The model under review builds one solid part; all positions refer to its coordinate system, in mm. A direction names the side the tool comes from. Give positions to 0.01 mm unless a question says otherwise; leave off trailing zeros. Loops run counter-clockwise (first coordinate to the right, second up) from the corner with the lowest first, then second, coordinate; pieces in that order, holes last. Notation, with made-up numbers: M 69.5,-2 L 123.5,-2 A36 ccw 123.5,35 Z; hole C 74,18 d5. An arc over 180 degrees is marked long. One line per item, written item: value. Start each with the question number.
Q1. For pin 1 (2 mm diameter, centred on x = 67.5, y = 268.5, fed in from +Z); pin 2 (8 mm diameter, centred on x = -8, y = 122.5, fed in from -Z), all flat-tipped, find the tip position at first contact; note any pin that passes through.
Q2. Mouldability with a two-part tool opening along X and no side actions: class faces 3 (the face through (-289, -6, 10)), 4 (the face through (288, -6, 10)), 5 (the face through (-4, -424, 10)) as released by +X, released by -X, zero draft, split by the parting line, or undercut.
Q3. To check wall thickness, follow line 1 along X through (y, z) = (299.5, 14.75); line 2 along Y through (x, z) = (-0.5, 10.5); line 3 along Z through (x, y) = (-61, 304). State the ranges of each line that lie inside material, in increasing order. Write a range as from..to.
Q4. For faces 1 (the face through (-288, -6, 10)), 2 (the face through (289, -6, 10)), list the 3-axis set-ups (+Z, -Z, +X, -X, +Y, -Y) from which the entire face can be reached by the end or side of a thin tool; tool diameter is ignored.
Q5. We need section A-A on y = 242.5. Write out the cut boundary in (x, z), plus the area to 3 significant figures.
Q6. We need section B-B on z = 10. Write out the cut boundary in (x, y).
Q7. We need section C-C on x = -161. Write out the cut boundary in (y, z).
```python
from build123d import *

# Parameters (mm, degrees)
SKETCH_1_W      = 578
SKETCH_1_H      = 848
EXTRUDE_1_DEPTH = 20
SHELL_1_T       = -1


with BuildPart() as part:
    # 草图1 → 凸台-拉伸1 (new body)
    with BuildSketch(Plane.XY):
        Rectangle(SKETCH_1_W, SKETCH_1_H)
    extrude(amount=EXTRUDE_1_DEPTH)

    # 抽壳1
    shell_1_openings = [part.faces().sort_by_distance(p)[0] for p in [
        (0, 0, 20),
    ]]
    offset(amount=SHELL_1_T, openings=shell_1_openings, kind=Kind.INTERSECTION)


solid = part.part
```
Solved:
1. pin 1: z = 1
1. pin 2: z = 0
2. face 3: released by -X
2. face 4: undercut
2. face 5: zero draft
3. line 1: -289..-288, 288..289
3. line 2: -424..-423, 423..424
3. line 3: 0..1
4. face 1: +Z
4. face 2: +Z, -Z, +X, +Y, -Y
5. outline: M -289,0 L 289,0 L 289,20 L 288,20 L 288,1 L -288,1 L -288,20 L -289,20 Z
5. area: 616 mm2
6. outline: M -289,-424 L 289,-424 L 289,424 L -289,424 Z; hole M -288,-423 L 288,-423 L 288,423 L -288,423 Z
7. outline: M -424,0 L 424,0 L 424,20 L 423,20 L 423,1 L -423,1 L -423,20 L -424,20 Z
